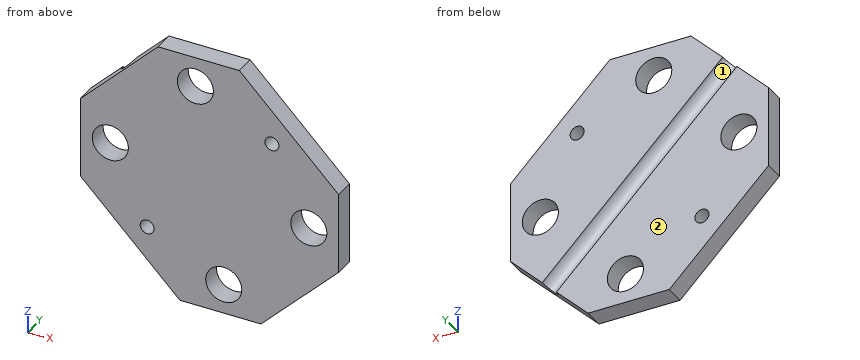
```python
from build123d import *

# Parameters (mm, degrees)
SKETCH1_R           = 4.5
BOSS_EXTRUDE1_DEPTH = 5
CUT_EXTRUDE1_REACH  = 80.329
CUT_EXTRUDE3_REACH  = 59.217
SKETCH6_R           = 1.75


with BuildPart() as part:
    # Sketch1 → Boss-Extrude1 (new body)
    with BuildSketch(Plane(origin=(0, 0, 0), x_dir=(1, 0, 0), z_dir=(0, 1, 0))):
        Polygon((-40.303943114, 15.555205773), (-15.555205773, 40.303943114), (4.694794227, 40.303943114), (24.042773974, 20.955963368), (24.042773974, 0.705963368), (-0.705963368, -24.042773974), (-20.955963368, -24.042773974), (-40.303943114, -4.694794227), align=None)
        with Locations(Location((-11.666118476, -16.618152771, 0), (0, 0, 270))):
            Circle(SKETCH1_R, mode=Mode.SUBTRACT)
        with Locations(Location((16.618152771, 11.666118476, 0), (0, 0, 270))):
            Circle(SKETCH1_R, mode=Mode.SUBTRACT)
        with Locations(Location((-4.595050664, 32.879321912, 0), (0, 0, 270))):
            Circle(SKETCH1_R, mode=Mode.SUBTRACT)
        with Locations(Location((-32.879321912, 4.595050664, 0), (0, 0, 270))):
            Circle(SKETCH1_R, mode=Mode.SUBTRACT)
    extrude(amount=BOSS_EXTRUDE1_DEPTH)

    # Sketch4 → Cut-Extrude1 (cut, up to next)
    with BuildSketch(Plane(origin=(22.499368671, 0, -22.499368671), x_dir=(-0.7071067811865465, 0, -0.7071067811865487), z_dir=(0.7071067811865487, 0, -0.7071067811865465)), mode=Mode.PRIVATE) as cut_extrude1_sk1:
        with BuildLine():
            Line((13.998382969, 5), (8.998382969, 5))
            ThreePointArc((8.998382969, 5), (11.498382969, 2.5), (13.998382969, 5))
        make_face()
    cut_extrude1_tool1 = extrude(cut_extrude1_sk1.sketch, amount=-CUT_EXTRUDE1_REACH, mode=Mode.PRIVATE) & part.part
    add(cut_extrude1_tool1.solids().sort_by_distance((14.368784, 3.938967, -30.629953))[0], mode=Mode.SUBTRACT)

    # Sketch6 → Cut-Extrude3 (cut, up to next)
    with BuildSketch(Plane(origin=(0, 5, 0), x_dir=(1, 0, 0), z_dir=(0, 1, 0)), mode=Mode.PRIVATE) as cut_extrude3_sk1:
        with Locations(Location((-23.686933757, 23.686933757, 0), (0, 0, 270))):
            Circle(SKETCH6_R)
    cut_extrude3_tool1 = extrude(cut_extrude3_sk1.sketch, amount=-CUT_EXTRUDE3_REACH, mode=Mode.PRIVATE) & part.part
    # Sketch6 → Cut-Extrude3 (cut, up to next)
    with BuildSketch(Plane(origin=(0, 5, 0), x_dir=(1, 0, 0), z_dir=(0, 1, 0)), mode=Mode.PRIVATE) as cut_extrude3_sk2:
        with Locations(Location((7.425764616, -7.425764616, 0), (0, 0, 270))):
            Circle(SKETCH6_R)
    cut_extrude3_tool2 = extrude(cut_extrude3_sk2.sketch, amount=-CUT_EXTRUDE3_REACH, mode=Mode.PRIVATE) & part.part
    add(cut_extrude3_tool1.solids().sort_by_distance((-23.686934, 5, -23.686934))[0], mode=Mode.SUBTRACT)
    add(cut_extrude3_tool2.solids().sort_by_distance((7.425765, 5, 7.425765))[0], mode=Mode.SUBTRACT)


solid = part.part
```
Source: CAD feature listing. Evaluate the final solid. Frame: model axes, mm. Face numbers are marked on the shaded views. Give positions to 0.01 mm unless a question says otherwise; leave off trailing zeros. Loops run counter-clockwise (first coordinate to the right, second up) from the corner with the lowest first, then second, coordinate; pieces in that order, holes last. Notation, with made-up numbers: M -26,-22.5 L 2,-22.5 A12 ccw 2,-5.5 Z; hole C -29.75,17 d4. An arc over 180 degrees is marked long. Put each result on its own line as item: value.
Q1. Section B-B (z = -34). Return the cut outline in (x, y).
Response values:
outline: M -21.86,0 L -8.95,0 L -8.95,5 L -21.86,5 Z; M -0.24,0 L 11,0 L 11,5 L -0.24,5 Z
Q2. Line query: probe 1 along X at (y, z) = (2.4, -8.5); probe 2 along Z at (x, y) = (-15.5, 4.5); probe 3 along Z at (x, y) = (-12, 1). Output: solid intervals per line, ascending. Write a range as [from, to].
Response values:
probe 1: x = [-40.3, -35.12], [-30.64, 13.42], [19.82, 24.04]
probe 2: z = [-40.3, -4.23], [2.7, 14.26], [18.97, 24.04]
probe 3: z = [-40.3, 12.13], [21.11, 24.04]
Q3. Pin query (flat end, axial travel): P1, Ø5.5, axis at x = -4.6, z = -32.88, coming from the +Y side; P2, Ø3, axis at y = 2, z = 13, coming from the +X side; P3, Ø1.5, axis at x = 6.5, y = 4.5, coming from the -Z side; P4, Ø3, axis at y = 3, z = -31, coming from the -X side. Return the tip coordinate at first contact, or that it passes through.
Response values:
P1: passes through
P2: stops at x = 11.84
P3: stops at z = -39.25
P4: stops at x = -26.36
Q4. Mould query, pull axis Z, two halves, no side actions, for the marked faces 1 and 2. Classes: released by +Z, released by -Z, zero draft, split by the parting line, or undercut.
Response values:
face 1: undercut
face 2: zero draft
Q5. Section A-A (y = 3.85). Return the cut outline in (x, z).
Response values:
outline: M -40.3,-15.56 L -15.56,-40.3 L 4.69,-40.3 L 12.8,-32.2 L -32.2,12.8 L -40.3,4.69 Z; M -29.06,15.94 L 15.94,-29.06 L 24.04,-20.96 L 24.04,-0.71 L -0.71,24.04 L -20.96,24.04 Z; hole C -32.88,-4.6 d9; hole C -23.69,-23.69 d3.5; hole C -11.67,16.62 d9; hole C -4.6,-32.88 d9; hole C 7.43,7.43 d3.5; hole C 16.62,-11.67 d9
